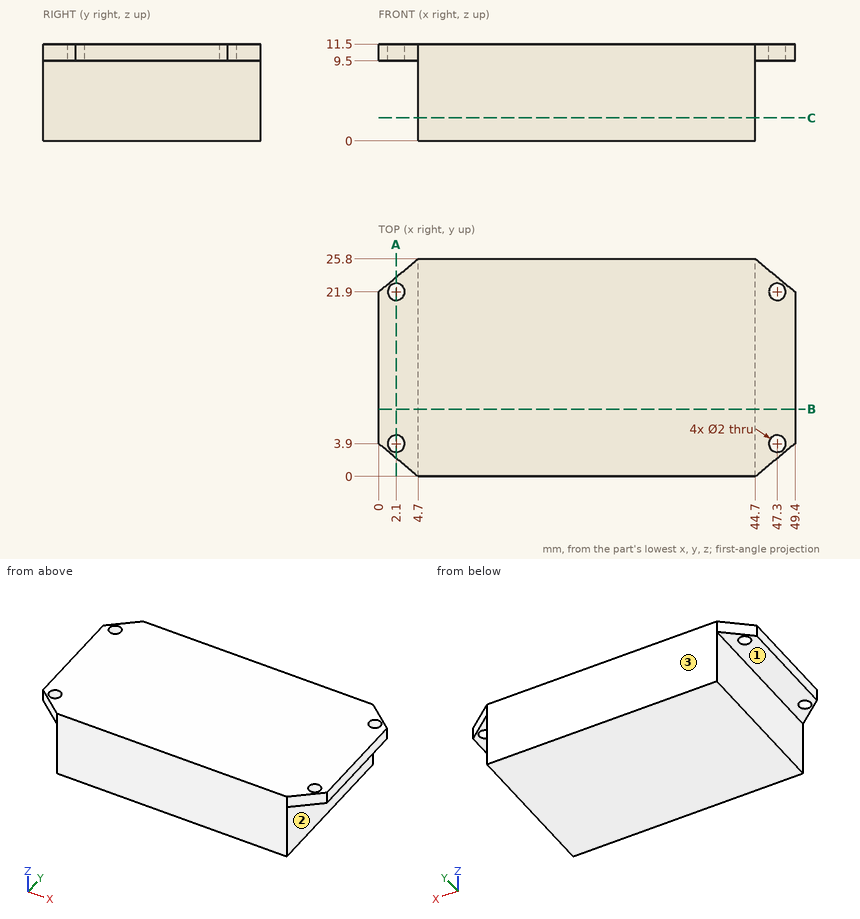
Can you work these out from the drawing? Everything is in mm from the part's minimum corner. A direction names the side the tool comes from. Coordinates: 2 decimals unless noted, no trailing zeros. Loops run counter-clockwise (first coordinate to the right, second up) from the corner with the lowest first, then second, coordinate; pieces in that order, holes last.
1) Imagine slicing it at C-C (z = 2.75). List the corners of the cut face in (x, y) for me.
Reported:
outline: (4.7, 0) - (44.7, 0) - (44.7, 25.8) - (4.7, 25.8) - close
2) Which directions (+Z, -Z, +X, -X, +Y, -Y) give clear straight access to the entire face, cutting with the end or side of a thin tool? Please do the marked faces 1, 2 and 3.
Reported:
face 1: -Z, -X, +Y, -Y
face 2: -Z, +X, +Y, -Y
face 3: +Z, -Z, +X, -X, +Y
3) Imagine slicing it at A-A (x = 2.1). List the corners of the cut face in (y, z) for me, and give its area (3 significant figures).
Reported:
outline: (2.16, 9.5) - (2.9, 9.5) - (2.9, 11.5) - (2.16, 11.5) - close; (4.9, 9.5) - (20.9, 9.5) - (20.9, 11.5) - (4.9, 11.5) - close; (22.9, 9.5) - (23.64, 9.5) - (23.64, 11.5) - (22.9, 11.5) - close
area: 35.0 mm2
4) Will these pins go through, and if not, where does the flat tip stop? pin 1 Ø2 at (y, z) = (17, 6) entering from -X; pin 2 Ø3 at (y, z) = (9.5, 6) entering from +X; pin 3 Ø5 at (x, y) = (47, 17) entering from -Z; pin 4 Ø4 at (x, y) = (1.5, 6.5) entering from -Z.
Reported:
pin 1: stops at x = 4.7
pin 2: stops at x = 44.7
pin 3: stops at z = 0
pin 4: stops at z = 9.5
5) Please list where these lines run through material, in increasing order: line 1 along Y through (x, z) = (2.1, 10.7); line 2 along X through (y, z) = (21.5, 8); line 3 along Z through (x, y) = (47, 2.75).
Reported:
line 1: y = 2.16 to 2.9, 4.9 to 20.9, 22.9 to 23.64
line 2: x = 4.7 to 44.7
line 3: z = 9.5 to 11.5
6) Imagine slicing it at B-B (y = 8). List the corners of the cut face in (x, z) for me, and give its area (3 significant figures).
Reported:
outline: (0, 9.5) - (4.7, 9.5) - (4.7, 0) - (44.7, 0) - (44.7, 9.5) - (49.4, 9.5) - (49.4, 11.5) - (0, 11.5) - close
area: 479 mm2
